Input: dimensioned drawing with shaded views. Units: mm. Origin: part minimum x, y, z. A direction names the side the tool comes from. Round coordinates to 2 decimals unless told otherwise and drop trailing zeros. Write each loop counter-clockwise with the first axis right and the second up, starting at its lowest first coordinate (ties: lowest second). Pieces come first, ordered by that corner, then holes. Notation, with made-up numbers: M 8,-5 L 58,-5 A33 cw 58,34 Z; hole C 82,-33.5 d11. An arc over 180 degrees is marked long. Answer as CSV lines item,"result". Start each with the question number.
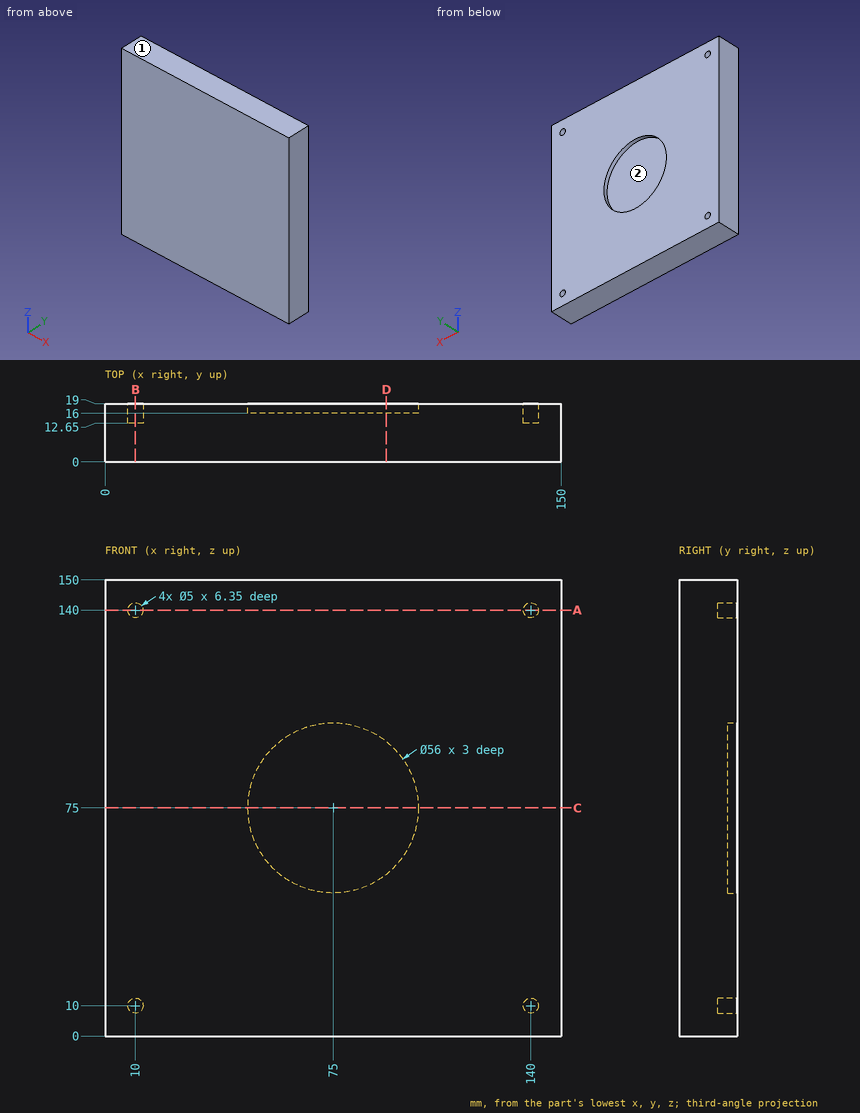
Item 1: Cut plane A-A, the plane z = 140. Return loops of the section in (x, y).
Item 2: Access query for the marked faces 1 and 2. Directions: +Z, -Z, +X, -X, +Y, -Y. A direction counts if a zero-diameter tool reaches every point of the face in a straight line with its end or side. Return the directions, or none.
Item 3: Pin query (flat end, axial travel): pin 1 Ø4 at (x, z) = (10, 10) entering from +Y. Return the tip coordinate at first contact, or that it passes through.
Item 4: Cut plane D-D, the plane x = 92.5. Return loops of the section in (y, z), plus the area to 3 significant figures.
Item 5: Line query: line 1 (Z direction, x = 10, y = 14.5); line 2 (Z direction, x = 75, y = 16.7). Output: solid intervals per line, ascending. Write a range as [from, to].
Item 6: Cut plane B-B, the plane x = 10. Return loops of the section in (y, z).
Item 7: Cut plane C-C, the plane z = 75. Return loops of the section in (x, y).
Results list:
1,outline,"M 0,0 L 150,0 L 150,19 L 142.5,19 L 142.5,12.65 L 137.5,12.65 L 137.5,19 L 12.5,19 L 12.5,12.65 L 7.5,12.65 L 7.5,19 L 0,19 Z"
2,face 1,"+Z, +X, -X, +Y, -Y"
2,face 2,"+Y"
3,pin 1,"y = 12.65"
4,outline,"M 0,0 L 19,0 L 19,53.14 L 16,53.14 L 16,96.86 L 19,96.86 L 19,150 L 0,150 Z"
4,area,"2,720 mm²"
5,line 1,"[0, 7.5], [12.5, 137.5], [142.5, 150]"
5,line 2,"[0, 47], [103, 150]"
6,outline,"M 0,0 L 19,0 L 19,7.5 L 12.65,7.5 L 12.65,12.5 L 19,12.5 L 19,137.5 L 12.65,137.5 L 12.65,142.5 L 19,142.5 L 19,150 L 0,150 Z"
7,outline,"M 0,0 L 150,0 L 150,19 L 103,19 L 103,16 L 47,16 L 47,19 L 0,19 Z"
